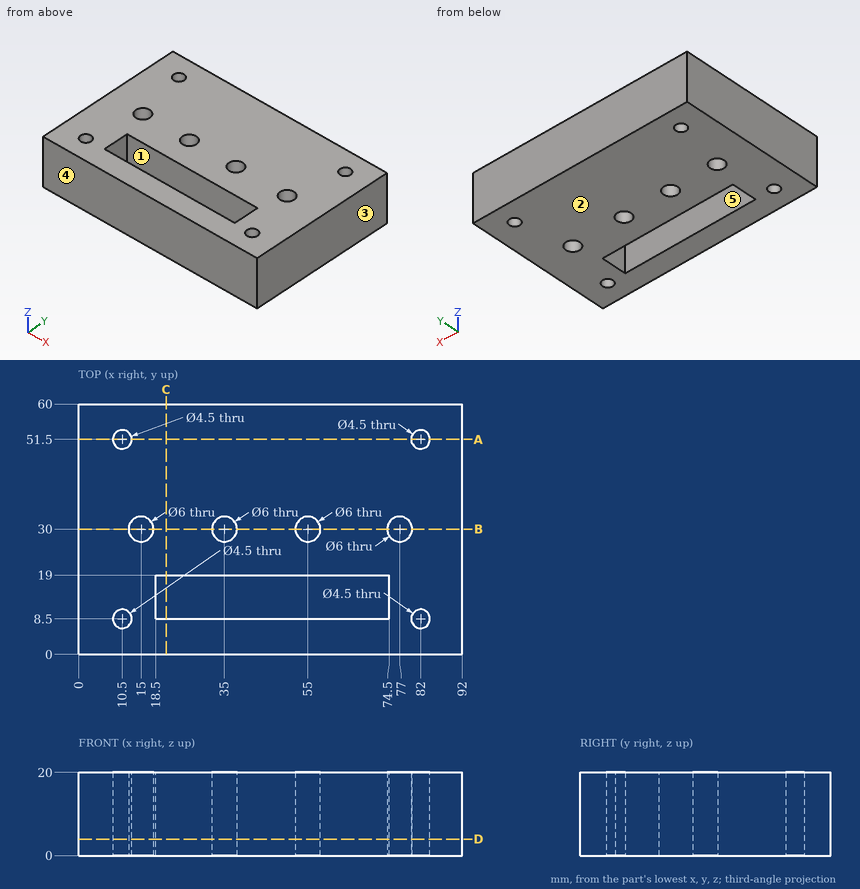
Geometry: see drawing. Coordinates: mm, zero at the bounding-box minimum. A direction names the side the tool comes from. Coordinates: 2 decimals unless noted, no trailing zeros. Write each loop counter-clockwise with the first axis right and the second up, starting at its lowest first coordinate (ties: lowest second). Pieces come first, ordered by that corner, then holes.
1) Section A-A on y = 51.5. Output: boundary loops of the cut face in (x, z).
2) Section B-B on y = 30. Output: boundary loops of the cut face in (x, z), and give its area (3 significant figures).
3) Section C-C on x = 21. Output: boundary loops of the cut face in (y, z).
4) Mould query, pull axis X, two halves, no side actions, for the marked faces 3, 4 and 5. Classes: pulls with the +X half, pulls with the -X half, needs draft (parallel to the pull), parting line crosses it, or undercut.
5) Material intervals for line 1 along Y through (x, z) = (55, 6.25); line 2 along Y through (x, z) = (77, 6); line 3 along Y through (x, z) = (57.5, 5.5), sorted ascending.
6) Section D-D on z = 4. State how many separate pieces and enclosed holes the cut face has, and give its area (3 significant figures).
7) Set-up query: the marked faces 1 and 2. Return all of +Z, -Z, +X, -X, +Y, -Y with unobstructed straight access to the full face (end or side cutting, diameter ignored); none if empty.
Check result:
1. outline: (0, 0) - (8.25, 0) - (8.25, 20) - (0, 20) - close; (12.75, 0) - (79.75, 0) - (79.75, 20) - (12.75, 20) - close; (84.25, 0) - (92, 0) - (92, 20) - (84.25, 20) - close
2. outline: (0, 0) - (12, 0) - (12, 20) - (0, 20) - close; (18, 0) - (32, 0) - (32, 20) - (18, 20) - close; (38, 0) - (52, 0) - (52, 20) - (38, 20) - close; (58, 0) - (74, 0) - (74, 20) - (58, 20) - close; (80, 0) - (92, 0) - (92, 20) - (80, 20) - close
2. area: 1,360 mm2
3. outline: (0, 0) - (8.5, 0) - (8.5, 20) - (0, 20) - close; (19, 0) - (60, 0) - (60, 20) - (19, 20) - close
4. face 3: pulls with the +X half
4. face 4: needs draft
4. face 5: undercut
5. line 1: y = 0 to 8.5, 19 to 27, 33 to 60
5. line 2: y = 0 to 27, 33 to 60
5. line 3: y = 0 to 8.5, 19 to 28.34, 31.66 to 60
6. separate pieces: 1
6. enclosed holes: 9
6. area: 4,760 mm2
7. face 1: +Z, -Z
7. face 2: -Z, +X, -X, +Y, -Y
